Geometry: final body of the model. Coordinates: model frame, mm. A direction names the side the tool comes from. Give positions to 0.01 mm unless a question says otherwise; leave off trailing zeros. Order: outer loops, then holes, each group sorted by start corner. A loop starts at its lowest first (then second) coordinate and runs counter-clockwise, first axis right, second up. Notation, with made-up numbers: M -23,61.25 L -3,61.25 A21 cw -3,71.25 Z; hole C 27.25,11 d4. An arc over 180 degrees is marked long. Use CSV: the item, a comma, the result in double quotes.
```python
from build123d import *

# Parameters (mm, degrees)
ESQUISSE1_W             = 152.4
ESQUISSE1_H             = 12.7
BOSS_EXTRU_1_DEPTH      = 6.35
ESQUISSE2_R             = 2.38125
ENL_V_MAT_EXTRU_1_DEPTH = 154.060029074
SKETCH1_W               = 14.17076538
SKETCH1_H               = 3.175
CUT_REVOLVE1_ANGLE      = 180
SKETCH2_W               = 3.175
SKETCH2_H               = 3.683
CUT_EXTRUDE1_DEPTH      = 154.060029074


with BuildPart() as part:
    # Esquisse1 → Boss.-Extru.1 (new body)
    with BuildSketch(Plane.XY):
        with Locations((-76.2, 6.35)):
            Rectangle(ESQUISSE1_W, ESQUISSE1_H)
    extrude(amount=-BOSS_EXTRU_1_DEPTH)

    # Esquisse2 → Enlèv. mat.-Extru.1 (cut, through all)
    with BuildSketch(Plane.XY):
        with Locations((-146.05, 6.35)):
            Circle(ESQUISSE2_R)
        with Locations((-76.2, 6.35)):
            Circle(ESQUISSE2_R)
        with Locations((-6.35, 6.35)):
            Circle(ESQUISSE2_R)
        with BuildLine():
            Line((0, 12.7), (-6.35, 12.7))
            ThreePointArc((-6.35, 12.7), (-1.859871939, 10.840128061), (0, 6.35))
            Line((0, 6.35), (0, 12.7))
        make_face()
        with BuildLine():
            Line((0, 0), (0, 6.35))
            ThreePointArc((0, 6.35), (-1.859871939, 1.859871939), (-6.35, 0))
            Line((-6.35, 0), (0, 0))
        make_face()
        with BuildLine():
            ThreePointArc((-152.4, 6.35), (-150.540128061, 10.840128061), (-146.05, 12.7))
            Line((-146.05, 12.7), (-152.4, 12.7))
            Line((-152.4, 12.7), (-152.4, 6.35))
        make_face()
        with BuildLine():
            ThreePointArc((-146.05, 0), (-150.540128061, 1.859871939), (-152.4, 6.35))
            Line((-152.4, 6.35), (-152.4, 0))
            Line((-152.4, 0), (-146.05, 0))
        make_face()
    extrude(amount=-ENL_V_MAT_EXTRU_1_DEPTH, mode=Mode.SUBTRACT)

    # Sketch1 → Cut-Revolve1 (revolve, symmetric, cut)
    with BuildSketch(Plane(origin=(0, 6.35, 0), x_dir=(1, 0, 0), z_dir=(0, 1, 0))) as cut_revolve1_sk:
        Polygon((-150.5585, 1.5875), (-152.4, 1.5875), (-152.4, 4.7625), (-150.5585, 4.7625), (-148.717, 4.7625), (-148.717, 1.5875), align=None)
        with Locations((-159.48538269, 3.175)):
            Rectangle(SKETCH1_W, SKETCH1_H)
    cut_revolve1 = revolve(axis=Axis((-146.05, 6.35, -6.35), (0, 0, 1)), revolution_arc=CUT_REVOLVE1_ANGLE / 2, mode=Mode.SUBTRACT)
    cut_revolve1 = cut_revolve1 + revolve(cut_revolve1_sk.sketch, axis=Axis((-146.05, 6.35, -6.35), (0, 0, -1)), revolution_arc=CUT_REVOLVE1_ANGLE / 2, mode=Mode.SUBTRACT)

    # Mirror1: Cut-Revolve1 across plane
    add(cut_revolve1.mirror(Plane(origin=(-76.2, 0, 0), x_dir=(0, 0, 1), z_dir=(1, 0, 0))), mode=Mode.SUBTRACT)

    # Sketch2 → Cut-Extrude1 (cut, through all)
    with BuildSketch(Plane(origin=(0, 0, 0), x_dir=(0, 0, -1), z_dir=(1, 0, 0))):
        with Locations((3.175, 10.8585)):
            Rectangle(SKETCH2_W, SKETCH2_H)
    cut_extrude1 = extrude(amount=-CUT_EXTRUDE1_DEPTH, mode=Mode.SUBTRACT)

    # Mirror2: Cut-Extrude1 across plane
    add(cut_extrude1.mirror(Plane.ZX.offset(6.35)), mode=Mode.SUBTRACT)


solid = part.part
```
1. Pull-direction query (Z, two-part tool) for faces 5 (the face through (-77.3, 9.3, -4.762)), 6 (the face through (-77.3, 3.6, -6.35)), 7 (the face through (-78.58, 6.45, -3.13)); classes: +Z half, -Z half, draft (parallel to the pull), parting line (faces both ways), or undercut.
Answer:
face 5,"undercut"
face 6,"-Z half"
face 7,"draft"
2. Line query: line 1 (Z direction, x = -7, y = 9.25); line 2 (Y direction, x = -146.05, z = -3); line 3 (Y direction, x = -32.5, z = -3.25). Output: solid intervals per line, ascending.
Answer:
line 1,"-6.35 to -4.76, -1.59 to 0"
line 2,"3.68 to 3.97, 8.73 to 9.02"
line 3,"3.68 to 9.02"
3. Pin query (flat end, axial travel): pin 1 Ø1 at (y, z) = (11.5, -4.5) entering from -X; pin 2 Ø1 at (x, z) = (-69.5, -4) entering from -Y; pin 3 Ø1 at (x, z) = (-18.5, -4) entering from +Y. Return the tip coordinate at first contact, or that it passes through.
Answer:
pin 1,"x = -150.29"
pin 2,"y = 3.68"
pin 3,"y = 9.02"
4. Section A-A, the plane x = -76.2. Return the cut outline in (y, z), plus the area to 3 significant figures.
Answer:
outline,"M 0,-6.35 L 3.97,-6.35 L 3.97,0 L 0,0 L 0,-1.59 L 3.68,-1.59 L 3.68,-4.76 L 0,-4.76 Z; M 8.73,-6.35 L 12.7,-6.35 L 12.7,-4.76 L 9.02,-4.76 L 9.02,-1.59 L 12.7,-1.59 L 12.7,0 L 8.73,0 Z"
area,"27.0 mm2"
5. Reachability of faces 1 (the face through (-75, 3.683, -3)), 2 (the face through (-75, 9.017, -3)), 3 (the face through (-148.716, 6.291, -3.153)), 4 (the face through (-3.684, 6.409, -3.153)) from +Z, -Z, +X, -X, +Y, -Y: full face, straight path, thin tool, end or side. Return the list, or none.
Answer:
face 1,"+X, -X, -Y"
face 2,"+X, -X, +Y"
face 3,"-X"
face 4,"+X"
6. Section B-B, the plane x = -36. Return the cut outline in (y, z).
Answer:
outline,"M 0,-6.35 L 12.7,-6.35 L 12.7,-4.76 L 9.02,-4.76 L 9.02,-1.59 L 12.7,-1.59 L 12.7,0 L 0,0 L 0,-1.59 L 3.68,-1.59 L 3.68,-4.76 L 0,-4.76 Z"
